Could you check a few things on this model? Use its own coordinates, in mm. Coordinates: 2 decimals unless noted, no trailing zeros. Order: outer loops, then holes, each group sorted by start corner. A loop starts at its lowest first (then second) coordinate and runs counter-clockwise, first axis right, second up. Notation, with made-up numbers: (-5.75, -21) -> (33.25, -21) arc R13 cw to (33.25, 2) -> close; hole circle Ø4 at (43.5, -5). An arc over 180 degrees is marked (long way). Put each result on its own line as item: value. Start each with the question number.
Q1. If we section it at C-C (x = -11.75): Please give me the cut outline in (y, z).
Q2. Please list where these lines run through material, in increasing order: line 1 along Z through (x, y) = (2.5, 1.8); line 2 along X through (y, z) = (0.85, 26); line 3 along X through (y, z) = (0.6, -8).
Q3. Will these pins go through, and if not, where does the flat tip stop? pin 1 (0.6 mm diameter, centred on y = 1, z = 28.5, fed in from -X); pin 2 (0.6 mm diameter, centred on x = 0, y = 1, fed in from +Z).
Q4. If we section it at B-B (z = 8): Please give me the cut outline in (x, y), and give its area (3 significant figures).
Q5. If we section it at A-A (x = -0.25): Please give me the cut outline in (y, z).
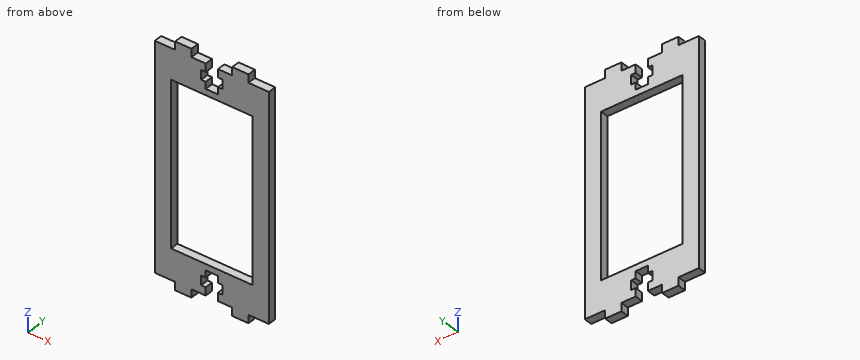
from build123d import *

# Parameters (mm, degrees)
SKETCH1_W           = 20
SKETCH1_H           = 40
BOSS_EXTRUDE1_DEPTH = 2
CUT_EXTRUDE2_DEPTH  = 2


with BuildPart() as part:
    # Sketch1 → Boss-Extrude1 (new body)
    with BuildSketch(Plane(origin=(0, 0, 0), x_dir=(1, 0, 0), z_dir=(0, 1, 0))):
        Polygon((-14, -27.5), (-9, -27.5), (-9, -29.5), (-5, -29.5), (-5, -27.5), (5, -27.5), (5, -29.5), (9, -29.5), (9, -27.5), (14, -27.5), (14, 27.5), (9, 27.5), (9, 29.5), (5, 29.5), (5, 27.5), (-5, 27.5), (-5, 29.5), (-9, 29.5), (-9, 27.5), (-14, 27.5), (-14, 14.5), (-14, -14.5), align=None)
        Rectangle(SKETCH1_W, SKETCH1_H, mode=Mode.SUBTRACT)
    extrude(amount=BOSS_EXTRUDE1_DEPTH)

    # Sketch4 → Cut-Extrude2 (cut)
    with BuildSketch(Plane(origin=(0, 2, 0), x_dir=(1, 0, 0), z_dir=(0, 1, 0))):
        Polygon((-1.5, 23.2), (-2.6, 23.2), (-2.6, 25.5), (-1.5, 25.5), (-1.5, 27.5), (1.5, 27.5), (1.5, 25.5), (2.6, 25.5), (2.6, 23.2), (1.5, 23.2), (1.5, 21.5), (-1.5, 21.5), align=None)
        Polygon((1.5, -25.5), (1.5, -27.5), (-1.5, -27.5), (-1.5, -25.5), (-2.6, -25.5), (-2.6, -23.2), (-1.5, -23.2), (-1.5, -21.5), (1.5, -21.5), (1.5, -23.2), (2.6, -23.2), (2.6, -25.5), align=None)
    extrude(amount=-CUT_EXTRUDE2_DEPTH, mode=Mode.SUBTRACT)


solid = part.part
The answers:
1. outline: (0, -27.5) -> (2, -27.5) -> (2, 27.5) -> (0, 27.5) -> close
2. line 1: -27.5 to -25.5, -23.2 to -20, 20 to 23.2, 25.5 to 27.5
2. line 2: -14 to -1.5, 1.5 to 14
2. line 3: -14 to -10, 10 to 14
3. pin 1: x = -9
3. pin 2: z = 21.5
4. outline: (-14, 0) -> (-10, 0) -> (-10, 2) -> (-14, 2) -> close; (10, 0) -> (14, 0) -> (14, 2) -> (10, 2) -> close
4. area: 16.0 mm^2
5. outline: (0, -21.5) -> (2, -21.5) -> (2, -20) -> (0, -20) -> close; (0, 20) -> (2, 20) -> (2, 21.5) -> (0, 21.5) -> close
